```python
from build123d import *

# Parameters (mm, degrees)
SKETCH1_W           = 63.9826
SKETCH1_H           = 57.9882
BOSS_EXTRUDE1_DEPTH = 1.5875
SKETCH2_R           = 0.513965226
SKETCH2_R_2         = 1.1049
SKETCH2_R_3         = 1.0414
CUT_EXTRUDE1_DEPTH  = 7.62
SKETCH3_R           = 1.905
CUT_EXTRUDE2_DEPTH  = 44.204412584
SKETCH4_W           = 17.78
SKETCH4_H           = 6.5532
CUT_EXTRUDE3_DEPTH  = 0.635
SKETCH5_W           = 35.0012
SKETCH5_H           = 34.9885
CUT_EXTRUDE4_DEPTH  = 44.204412584
CUT_EXTRUDE5_DEPTH  = 44.204412584
SKETCH7_R           = 1.1049
CUT_EXTRUDE6_DEPTH  = 44.204412584
FILLET1_R           = 2.54
FILLET2_R           = 2.54
FILLET5_R           = 2.54
FILLET6_R           = 2.54
SKETCH8_R           = 1.1049
CUT_EXTRUDE7_DEPTH  = 2.54


with BuildPart() as part:
    # Sketch1 → Boss-Extrude1 (new body)
    with BuildSketch(Plane(origin=(0, 0, 0), x_dir=(1, 0, 0), z_dir=(0, 1, 0))):
        Rectangle(SKETCH1_W, SKETCH1_H)
    extrude(amount=BOSS_EXTRUDE1_DEPTH)

    # Sketch2 → Cut-Extrude1 (cut)
    with BuildSketch(Plane(origin=(0, 1.5875, 0), x_dir=(1, 0, 0), z_dir=(0, 1, 0))):
        with Locations(Location((0, 0, 0), (0, 0, 270))):
            Circle(SKETCH2_R)
        with Locations(Location((-23.495, -23.495, 0), (0, 0, 270))):
            Circle(SKETCH2_R_2)
        with Locations(Location((23.495, -23.495, 0), (0, 0, 270))):
            Circle(SKETCH2_R_2)
        with Locations(Location((-23.495, 23.495, 0), (0, 0, 270))):
            Circle(SKETCH2_R_2)
        with Locations(Location((23.495, 23.495, 0), (0, 0, 270))):
            Circle(SKETCH2_R_2)
        with Locations(Location((-5.0927, 19.939, 0), (0, 0, 270))):
            Circle(SKETCH2_R_3)
        with Locations(Location((5.0927, 19.939, 0), (0, 0, 270))):
            Circle(SKETCH2_R_3)
        with Locations(Location((5.0927, -19.939, 0), (0, 0, 270))):
            Circle(SKETCH2_R_3)
        with Locations(Location((-5.0927, -19.939, 0), (0, 0, 270))):
            Circle(SKETCH2_R_3)
    extrude(amount=-CUT_EXTRUDE1_DEPTH, mode=Mode.SUBTRACT)

    # Sketch3 → Cut-Extrude2 (cut, through all)
    with BuildSketch(Plane(origin=(0, 1.5875, 0), x_dir=(1, 0, 0), z_dir=(0, 1, 0))):
        with Locations(Location((0, 19.939, 0), (0, 0, 270))):
            Circle(SKETCH3_R)
        with BuildLine():
            Line((16.47985425, -9.525), (16.47985425, 9.525))
            ThreePointArc((16.47985425, 9.525), (19.05, 12.09514575), (21.62014575, 9.525))
            Line((21.62014575, 9.525), (21.62014575, -9.525))
            ThreePointArc((21.62014575, -9.525), (19.05, -12.09514575), (16.47985425, -9.525))
        make_face()
        with BuildLine():
            Line((-20.3835, -13.375), (-20.3835, -18.375))
            ThreePointArc((-20.3835, -18.375), (-20.955, -18.9465), (-21.5265, -18.375))
            Line((-21.5265, -18.375), (-21.5265, -13.375))
            ThreePointArc((-21.5265, -13.375), (-20.955, -12.8035), (-20.3835, -13.375))
        make_face()
    extrude(amount=-CUT_EXTRUDE2_DEPTH, mode=Mode.SUBTRACT)

    # Sketch4 → Cut-Extrude3 (cut)
    with BuildSketch(Plane(origin=(0, 1.5875, 0), x_dir=(1, 0, 0), z_dir=(0, 1, 0))):
        with Locations((24.7269, -16.8021)):
            Rectangle(SKETCH4_W, SKETCH4_H)
        with Locations((24.7269, 16.8021)):
            Rectangle(SKETCH4_W, SKETCH4_H)
    extrude(amount=-CUT_EXTRUDE3_DEPTH, mode=Mode.SUBTRACT)

    # Sketch5 → Cut-Extrude4 (cut, through all)
    with BuildSketch(Plane(origin=(0, 1.5875, 0), x_dir=(1, 0, 0), z_dir=(0, 1, 0))):
        with Locations((-2.1463, 0)):
            Rectangle(SKETCH5_W, SKETCH5_H)
    extrude(amount=-CUT_EXTRUDE4_DEPTH, mode=Mode.SUBTRACT)

    # Sketch6 → Cut-Extrude5 (cut, through all)
    with BuildSketch(Plane(origin=(0, 1.5875, 0), x_dir=(1, 0, 0), z_dir=(0, 1, 0))):
        with BuildLine():
            Line((-7.452592056, -17.49425), (-18.430007944, -17.49425))
            ThreePointArc((-18.430007944, -17.49425), (-19.013249676, -18.054409326), (-19.2278, -18.8341))
            ThreePointArc((-19.2278, -18.8341), (-18.781430735, -19.911730735), (-17.7038, -20.3581))
            Line((-17.7038, -20.3581), (-8.1788, -20.3581))
            ThreePointArc((-8.1788, -20.3581), (-6.701554692, -19.208696183), (-7.452592056, -17.49425))
        make_face()
        with BuildLine():
            Line((-18.430007944, -17.49425), (-19.6469, -17.49425))
            Line((-19.6469, -17.49425), (-19.6469, -18.8341))
            Line((-19.6469, -18.8341), (-19.2278, -18.8341))
            ThreePointArc((-19.2278, -18.8341), (-19.013249676, -18.054409326), (-18.430007944, -17.49425))
        make_face()
        with BuildLine():
            Line((-22.6568, 6.8834), (-22.6568, -8.9916))
            ThreePointArc((-22.6568, -8.9916), (-21.431305697, -10.537274003), (-19.6469, -9.696535806))
            Line((-19.6469, -9.696535806), (-19.6469, 7.588335806))
            ThreePointArc((-19.6469, 7.588335806), (-21.431305697, 8.429074003), (-22.6568, 6.8834))
        make_face()
        with BuildLine():
            Line((14.269902317, -17.49425), (7.857194183, -17.49425))
            ThreePointArc((7.857194183, -17.49425), (6.780339401, -18.977660877), (8.142735041, -20.20403854))
            Line((8.142735041, -20.20403854), (13.98436146, -20.20403854))
            ThreePointArc((13.98436146, -20.20403854), (14.953054291, -19.802792832), (15.3543, -18.8341))
            ThreePointArc((15.3543, -18.8341), (15.049233525, -17.972253674), (14.269902317, -17.49425))
        make_face()
        with BuildLine():
            Line((14.904303176, -17.49425), (14.269902317, -17.49425))
            ThreePointArc((14.269902317, -17.49425), (15.049233525, -17.972253674), (15.3543, -18.8341))
            Line((15.3543, -18.8341), (15.3543, -17.49425))
            Line((15.3543, -17.49425), (14.904303176, -17.49425))
        make_face()
        with BuildLine():
            ThreePointArc((8.142735041, 20.20403854), (6.780339401, 18.977660877), (7.857194183, 17.49425))
            Line((7.857194183, 17.49425), (14.269902317, 17.49425))
            ThreePointArc((14.269902317, 17.49425), (15.049233525, 17.972253674), (15.3543, 18.8341))
            ThreePointArc((15.3543, 18.8341), (14.953054291, 19.802792832), (13.98436146, 20.20403854))
            Line((13.98436146, 20.20403854), (8.142735041, 20.20403854))
        make_face()
        with BuildLine():
            ThreePointArc((15.3543, 18.8341), (15.049233525, 17.972253674), (14.269902317, 17.49425))
            Line((14.269902317, 17.49425), (14.904303176, 17.49425))
            Line((14.904303176, 17.49425), (15.3543, 17.49425))
            Line((15.3543, 17.49425), (15.3543, 18.8341))
        make_face()
    extrude(amount=-CUT_EXTRUDE5_DEPTH, mode=Mode.SUBTRACT)

    # Sketch7 → Cut-Extrude6 (cut, through all)
    with BuildSketch(Plane(origin=(0, 1.5875, 0), x_dir=(1, 0, 0), z_dir=(0, 1, 0))):
        with Locations(Location((-29.1465, -15.875, 0), (0, 0, 270))):
            Circle(SKETCH7_R)
        with Locations(Location((-29.1465, 17.145, 0), (0, 0, 270))):
            Circle(SKETCH7_R)
    extrude(amount=-CUT_EXTRUDE6_DEPTH, mode=Mode.SUBTRACT)

    # Fillet1
    fillet1_edges = [part.edges().sort_by_distance(p)[0] for p in [
        (-19.6469, 0.79375, -7.588335806),
        (-19.6469, 0.79375, 9.696535806),
    ]]
    fillet(fillet1_edges, radius=FILLET1_R)

    # Fillet2
    fillet2_edges = [part.edges().sort_by_distance(p)[0] for p in [
        (-7.452592056, 0.79375, 17.49425),
    ]]
    fillet(fillet2_edges, radius=FILLET2_R)

    # Fillet5
    fillet5_edges = [part.edges().sort_by_distance(p)[0] for p in [
        (7.857194183, 0.79375, 17.49425),
    ]]
    fillet(fillet5_edges, radius=FILLET5_R)

    # Fillet6
    fillet6_edges = [part.edges().sort_by_distance(p)[0] for p in [
        (7.857194183, 0.79375, -17.49425),
    ]]
    fillet(fillet6_edges, radius=FILLET6_R)

    # Sketch8 → Cut-Extrude7 (cut)
    with BuildSketch(Plane(origin=(0, 0.9525, 0), x_dir=(1, 0, 0), z_dir=(0, 1, 0))):
        with Locations(Location((19.3167, 15.2273, 0), (0, 0, 270))):
            Circle(SKETCH8_R)
        with Locations(Location((19.3167, -15.2273, 0), (0, 0, 270))):
            Circle(SKETCH8_R)
    extrude(amount=-CUT_EXTRUDE7_DEPTH, mode=Mode.SUBTRACT)


solid = part.part
```
Model file for the job. Use its own axes, mm. A direction names the side the tool comes from. Give positions to 0.01 mm unless a question says otherwise; leave off trailing zeros. Loops run counter-clockwise (first coordinate to the right, second up) from the corner with the lowest first, then second, coordinate; pieces in that order, holes last. Notation, with made-up numbers: (66.5, 81.5) -> (91.5, 81.5) arc R12 ccw to (91.5, 97.5) -> close; hole circle Ø11 at (66.25, -18). An arc over 180 degrees is marked (long way). Write each question's results on one line, items separated by ' | '.
(1) Probe line 1 along X through (y, z) = (0.1, -2.5); line 2 along Z through (x, y) = (10.5, 0.8); line 3 along Z through (x, y) = (-24.5, 1.3). List the from-to ranges inside material, lowest first.
Geometry results:
line 1: x = -31.99 to -22.66, 15.35 to 16.48, 21.62 to 31.99 | line 2: z = -28.99 to -20.2, 20.2 to 28.99 | line 3: z = -28.99 to -23.95, -23.04 to 23.04, 23.95 to 28.99
(2) Cut at A-A on x = -11.5. List the corners of the cut face in (y, z).
Geometry results:
outline: (0, -28.99) -> (1.59, -28.99) -> (1.59, -17.49) -> (0, -17.49) -> close; (0, 20.36) -> (1.59, 20.36) -> (1.59, 28.99) -> (0, 28.99) -> close
(3) Cut at D-D on x = 27. List the corners of the cut face in (y, z), and give its area (3 significant figures).
Geometry results:
outline: (0, -28.99) -> (1.59, -28.99) -> (1.59, -20.08) -> (0.95, -20.08) -> (0.95, -13.53) -> (1.59, -13.53) -> (1.59, 13.53) -> (0.95, 13.53) -> (0.95, 20.08) -> (1.59, 20.08) -> (1.59, 28.99) -> (0, 28.99) -> close | area: 83.7 mm²
(4) Cut at B-B on z = 4.5. List the corners of the cut face in (x, y).
Geometry results:
outline: (-31.99, 0) -> (-22.66, 0) -> (-22.66, 1.59) -> (-31.99, 1.59) -> close; (15.35, 0) -> (16.48, 0) -> (16.48, 1.59) -> (15.35, 1.59) -> close; (21.62, 0) -> (31.99, 0) -> (31.99, 1.59) -> (21.62, 1.59) -> close
(5) Flat gauge pins, fed straight in: pin 1 Ø2 at (x, z) = (21.5, 18) entering from +Y; pin 2 Ø2.5 at (x, z) = (0, -19.939) entering from -Y. Where does each tip first touch, or does it go through?
Geometry results:
pin 1: stops at y = 0.95 | pin 2: passes through
(6) Tool access for faces 1 (the cylindrical face through (-22.34, 0.8, 9.94)), 2 (the flat face through (24, 0.952, -17)), 3 (the flat face through (-8, 1.588, -20)): list every direction of +Z, -Z, +X, -X, +Y, -Y with a clear straight run to the whole face (end or side of a thin tool).
Geometry results:
face 1: +Y, -Y | face 2: +X, +Y | face 3: +Z, -Z, +X, -X, +Y
(7) Pull direction X, two halves, no side cores. Call faces 4 (the flat face through (0, 0, 19)), 5 (the flat face through (15.354, 1, 0)): released by +X, released by -X, zero draft, split by the parting line, or undercut.
Geometry results:
face 4: zero draft | face 5: undercut
(8) Cut at C-C on x = 0. List the corners of the cut face in (y, z).
Geometry results:
outline: (0, -28.99) -> (1.59, -28.99) -> (1.59, -21.84) -> (0, -21.84) -> close; (0, -18.03) -> (1.59, -18.03) -> (1.59, -17.49) -> (0, -17.49) -> close; (0, 17.49) -> (1.59, 17.49) -> (1.59, 28.99) -> (0, 28.99) -> close
